from build123d import *

# Parameters (mm, degrees)
SKETCH_1_W      = 22.5
SKETCH_1_H      = 11
SKETCH_1_W_2    = 4
SKETCH_1_H_2    = 4
SKETCH_1_R      = 1.25
EXTRUDE_1_DEPTH = 1
SKETCH_2_W      = 22.5
SKETCH_2_H      = 10
EXTRUDE_2_DEPTH = 5.5


with BuildPart() as part:
    # Эскиз1 → Бобышка-Вытянуть1 (new body)
    # profile 1 of 3: a face of its own
    with BuildSketch(Plane(origin=(0, 0, 0), x_dir=(1, 0, 0), z_dir=(0, 1, 0))):
        Rectangle(SKETCH_1_W, SKETCH_1_H)
    # profile 2 of 3: a face of its own
    with BuildSketch(Plane(origin=(0, 0, 0), x_dir=(1, 0, 0), z_dir=(0, 1, 0))):
        with Locations((-13.25, 0)):
            Rectangle(SKETCH_1_W_2, SKETCH_1_H_2)
        with Locations(Location((-13.25, 0, 0), (0, 0, 270))):
            Circle(SKETCH_1_R, mode=Mode.SUBTRACT)
    # profile 3 of 3: a face of its own
    with BuildSketch(Plane(origin=(0, 0, 0), x_dir=(1, 0, 0), z_dir=(0, 1, 0))):
        with Locations((13.25, 0)):
            Rectangle(SKETCH_1_W_2, SKETCH_1_H_2)
        with Locations(Location((13.25, 0, 0), (0, 0, 270))):
            Circle(SKETCH_1_R, mode=Mode.SUBTRACT)
    extrude(amount=EXTRUDE_1_DEPTH)

    # Эскиз2 → Бобышка-Вытянуть2 (add)
    with BuildSketch(Plane(origin=(0, 1, 0), x_dir=(1, 0, 0), z_dir=(0, 1, 0))):
        Rectangle(SKETCH_2_W, SKETCH_2_H)
    extrude(amount=EXTRUDE_2_DEPTH)


solid = part.part
Here's how the part is built. I have some questions about the finished solid (model axes, mm). A direction names the side the tool comes from. Round coordinates to 2 decimals unless told otherwise and drop trailing zeros. Write each loop counter-clockwise with the first axis right and the second up, starting at its lowest first coordinate (ties: lowest second). Pieces come first, ordered by that corner, then holes.
1. I need wall thicknesses on L1, parallel to X at y = 0.4, z = 0; L2, parallel to X at y = 0.75, z = -1; L3, parallel to Z at x = -4.5, y = 1.25. Which ranges of each line are inside material? Lowest first, please.
2. Will these pins go through, and if not, where does the flat tip stop? pin 1 Ø1.6 at (x, y) = (3.5, 5) entering from -Z; pin 2 Ø0.8 at (x, y) = (-12.5, 0.5) entering from +Z; pin 3 Ø3 at (x, z) = (13.25, 0) entering from +Y.
3. Suppose I cut it at C-C (x = -2.5). List the corners of the cut face in (y, z) for me.
4. If we mould it in two halves opening along X, with no side actions, what happens to faces 1 (the flat face through (15.25, 0.5, 0)), 2 (the flat face through (12, 1, -1)), 3 (the cylindrical face through (-12.01, 0.49, -0.16))? For each: released by +X, released by -X, zero draft, split by the parting line, or undercut.
5. Suppose I cut it at D-D (y = 5.5). List the corners of the cut face in (x, z) for me.
6. Suppose I cut it at A-A (z = -0.75). List the corners of the cut face in (x, y) for me, and give its area (3 significant figures).
7. For faces 4 (the flat face through (-13.3, 0.5, 2)), 5 (the flat face through (0, 4, -5)), 6 (the flat face through (13.2, 0.5, 2)), 7 (the flat face through (13.2, 0.5, -2)), 8 (the flat face through (-12, 1, -1)), which set-ups out of +Z, -Z, +X, -X, +Y, -Y let a thin tool reach every point of the face, with its end or its side?
8. Suppose I cut it at B-B (x = -13.25). List the corners of the cut face in (y, z) for me.
Answer sheet:
1. L1: x = -15.25 to -14.5, -12 to 12, 14.5 to 15.25
1. L2: x = -15.25 to -14, -12.5 to 12.5, 14 to 15.25
1. L3: z = -5 to 5
2. pin 1: stops at z = -5
2. pin 2: stops at z = 2
2. pin 3: stops at y = 1
3. outline: (0, -5.5) - (1, -5.5) - (1, -5) - (6.5, -5) - (6.5, 5) - (1, 5) - (1, 5.5) - (0, 5.5) - close
4. face 1: released by +X
4. face 2: zero draft
4. face 3: undercut
5. outline: (-11.25, -5) - (11.25, -5) - (11.25, 5) - (-11.25, 5) - close
6. outline: (-15.25, 0) - (-14.25, 0) - (-14.25, 1) - (-15.25, 1) - close; (-12.25, 0) - (12.25, 0) - (12.25, 1) - (11.25, 1) - (11.25, 6.5) - (-11.25, 6.5) - (-11.25, 1) - (-12.25, 1) - close; (14.25, 0) - (15.25, 0) - (15.25, 1) - (14.25, 1) - close
6. area: 150 mm2
7. face 4: +Z, -X, +Y, -Y
7. face 5: -Z, +X, -X, +Y
7. face 6: +Z, +X, +Y, -Y
7. face 7: -Z, +X, +Y, -Y
7. face 8: +Z, -Z, -X, +Y
8. outline: (0, -2) - (1, -2) - (1, -1.25) - (0, -1.25) - close; (0, 1.25) - (1, 1.25) - (1, 2) - (0, 2) - close
